```python
from build123d import *

# Parameters (mm, degrees)
F1_DEPTH    = 35.052
F1_FACE_W   = 38.608
F1_FACE_H   = 35.052
F1_FACE_W_2 = 37.592001
F2_DEPTH    = 1.016
F4_DEPTH    = 91.948


with BuildPart() as f1:
    # F0 (on Front) → F1 (new body)
    with BuildSketch(Plane.XZ):
        Polygon((0, 76.453999), (0, 0), (101.600006, 0), (101.600006, 76.453999), (64.008005, 76.453999), (64.008005, 50.546002), (38.608, 50.546002), (38.608, 76.453999), align=None)
    extrude(amount=F1_DEPTH)

    # F1_face (on face) → F2 (join)
    with BuildSketch(Plane(origin=(19.304, -17.526, 76.453999), x_dir=(1, 0, 0), z_dir=(0, 0, 1))):
        Rectangle(F1_FACE_W, F1_FACE_H)
        with Locations((63.500005, 0)):
            Rectangle(F1_FACE_W_2, F1_FACE_H)
    extrude(amount=-F2_DEPTH)


with BuildPart() as f4:
    # F3 (on face) → F4 (new body)
    with BuildSketch(Plane.XY.offset(76.453999)):
        Polygon((354.056151, 0), (354.056151, -101.6), (444.539875, -101.6), (444.539875, -47.334887), (531.121194, -47.334887), (522.471368, 0), (468.59476, 0), align=None)
    extrude(amount=-F4_DEPTH)


solid = f1.part
```
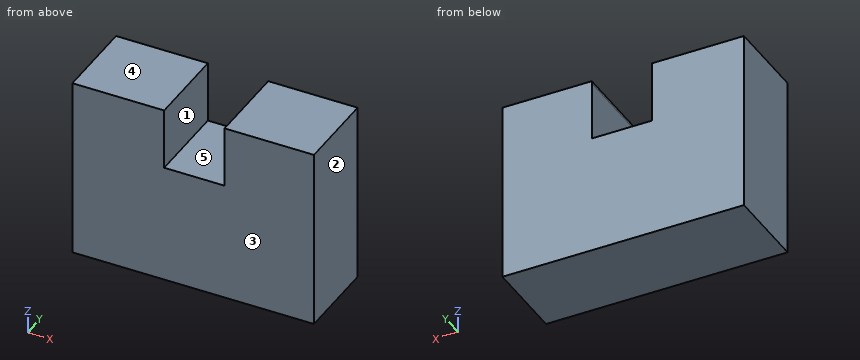
The model under review builds one solid part; all positions refer to its coordinate system, in mm. Face numbers are marked on the shaded views. A direction names the side the tool comes from. Round coordinates to 2 decimals unless told otherwise and drop trailing zeros. Write each loop counter-clockwise with the first axis right and the second up, starting at its lowest first coordinate (ties: lowest second). Pieces come first, ordered by that corner, then holes.
(1) We need section B-B on y = -18. Give the boundary of the cut face in (x, z), and give its area (3 significant figures).
(2) Insertion check: pin 1 (1 mm diameter, centred on y = -29.5, z = 61, fed in from -X); pin 2 (1 mm diameter, centred on x = 55.5, y = -27, fed in from +Z). Each pin has a flat end and moves straight along its axis. Give the tip position at first contact, or say it passes through.
(3) Machinability: for the marked faces 4 and 5, which of the approach directions +Z, -Z, +X, -X, +Y, -Y give a long, thin tool a straight path to every point of the face, cutting with its end or side? Answer none if there is none.
(4) We need section C-C on x = 58. Give the boundary of the cut face in (y, z).
(5) Wall thickness on L1, parallel to X at y = -24, z = 72.5; L2, parallel to Z at x = 61, y = -33: over which ranges is each line inside the solid? List them lowest first.
(6) Mouldability with a two-part tool opening along X and no side actions: class the marked faces 1, 2 and 3 as +X half, -X half, draft (parallel to the pull), parting line (faces both ways), or undercut.
(7) We need section A-A on z = 58. Give the boundary of the cut face in (x, y), and give its area (3 significant figures).
Findings below:
1. outline: (0, 0) - (101.6, 0) - (101.6, 76.45) - (64.01, 76.45) - (64.01, 50.55) - (38.61, 50.55) - (38.61, 76.45) - (0, 76.45) - close
1. area: 7,110 mm2
2. pin 1: stops at x = 0
2. pin 2: stops at z = 50.55
3. face 4: +Z, +X, -X, +Y, -Y
3. face 5: +Z, +Y, -Y
4. outline: (-35.05, 0) - (0, 0) - (0, 50.55) - (-35.05, 50.55) - close
5. L1: x = 0 to 38.61, 64.01 to 101.6
5. L2: z = 0 to 50.55
6. face 1: undercut
6. face 2: +X half
6. face 3: draft
7. outline: (0, -35.05) - (38.61, -35.05) - (38.61, 0) - (0, 0) - close; (64.01, -35.05) - (101.6, -35.05) - (101.6, 0) - (64.01, 0) - close
7. area: 2,670 mm2
